```python
from build123d import *

# Parameters (mm, degrees)
F1_DEPTH = 25
F2_R     = 2.5
F3_DEPTH = 4


with BuildPart() as f1:
    # F0 (on Top) → F1 (new body)
    with BuildSketch(Plane.XY):
        with BuildLine():
            Line((-9.697168, 7.274801), (-11.697168, 7.274801))
            ThreePointArc((-11.697168, 7.274801), (-13.111381, 6.689015), (-13.697168, 5.274801))
            Line((-13.697168, 5.274801), (-13.697168, -22.725199))
            Line((-13.697168, -22.725199), (-9.697168, -22.725199))
            Line((-9.697168, -22.725199), (-9.697168, 5.024801))
            ThreePointArc((-9.697168, 5.024801), (-9.623944, 5.201578), (-9.447168, 5.274801))
            Line((-9.447168, 5.274801), (20.302832, 5.274801))
            ThreePointArc((20.302832, 5.274801), (23.278921, 2.652814), (21.052832, -0.629937))
            ThreePointArc((21.052832, -0.629937), (20.512263, -0.98581), (20.302832, -1.598182))
            ThreePointArc((20.302832, -1.598182), (20.69046, -2.388752), (21.552832, -2.566428))
            ThreePointArc((21.552832, -2.566428), (25.262981, 2.904822), (20.302832, 7.274801))
            Line((20.302832, 7.274801), (-9.697168, 7.274801))
        make_face()
    extrude(amount=F1_DEPTH)

    # F2 (on face) → F3 (cut, through all)
    with BuildSketch(Plane(origin=(-13.697168, 0, 0), x_dir=(0, -1, 0), z_dir=(-1, 0, 0))):
        with Locations((12.725199, 12.5)):
            Circle(F2_R)
    extrude(amount=-F3_DEPTH, mode=Mode.SUBTRACT)


solid = f1.part
```
Design review of the part built by this model. Coordinates are the model's own, in mm. A direction names the side the tool comes from. Coordinates: 2 decimals unless noted, no trailing zeros. Write each loop counter-clockwise with the first axis right and the second up, starting at its lowest first coordinate (ties: lowest second). Pieces come first, ordered by that corner, then holes. Notation, with made-up numbers: M -30.75,-9 L -9.75,-9 A11 ccw -9.75,6 Z; hole C -32,45 d8. An arc over 180 degrees is marked long. Answer as a JSON object with one key per item and string values.
Item 1: Draft analysis for pull direction Y (two halves, no side actions). For faces 3 (the cylindrical face through (-11.725, -13.879, 10.282)), 4 (the flat face through (5, 7.275, 12)), 5 (the flat face through (-12, -22.725, 12)), 6 (the cylindrical face through (23.27, 2.71, 12.32)), state which applies: pulls with the +Y half, pulls with the -Y half, needs draft (parallel to the pull), parting line crosses it, or undercut.
Outcome:
{"face 3": "undercut", "face 4": "pulls with the +Y half", "face 5": "pulls with the -Y half", "face 6": "undercut"}
Item 2: Add section B-B, the plane x = 22. Give the boundary of the cut face in (y, z), and give its area (3 significant figures).
Outcome:
{"outline": "M -2.43,0 L -0.2,0 L -0.2,25 L -2.43,25 Z; M 4.75,0 L 6.98,0 L 6.98,25 L 4.75,25 Z", "area": "111 mm²"}
Item 3: Add section D-D, the plane z = 21.25. Give the boundary of the cut face in (x, y), and give its area (3 significant figures).
Outcome:
{"outline": "M -13.7,-22.73 L -9.7,-22.73 L -9.7,5.02 A0.25 cw -9.45,5.27 L 20.3,5.27 A3 cw 21.05,-0.63 A1 ccw 21.55,-2.57 A5 ccw 20.3,7.27 L -11.7,7.27 A2 ccw -13.7,5.27 Z", "area": "204 mm²"}
Item 4: Insertion check: pin 1 Ø7.5 at (x, z) = (5.5, 17.5) entering from -Y; pin 2 Ø4 at (x, y) = (-9.5, -15.5) entering from +Z; pin 3 Ø1 at (y, z) = (-5.5, 13.5) entering from +X; pin 4 Ø5 at (y, z) = (-1, 9) entering from +X. Each pin has a flat end and moves straight along its axis. Give the tip position at first contact, or say it passes through.
Outcome:
{"pin 1": "y = 5.27", "pin 2": "z = 25", "pin 3": "x = -9.7", "pin 4": "x = 25.24"}
Item 5: Machinability: for faces 1 (the flat face through (-9.697, -9, 12)), 2 (the flat face through (-10, -3, 0)), which of the approach directions +Z, -Z, +X, -X, +Y, -Y give a long, thin tool a straight path to every point of the face, cutting with its end or side? Answer none if there is none.
Outcome:
{"face 1": "+Z, -Z, -Y", "face 2": "-Z, +X, -X, +Y, -Y"}
Item 6: Add section A-A, the plane z = 12.5. Give the boundary of the cut face in (x, y).
Outcome:
{"outline": "M -13.7,-22.73 L -9.7,-22.73 L -9.7,-15.23 L -13.7,-15.23 Z; M -13.7,-10.23 L -9.7,-10.23 L -9.7,5.02 A0.25 cw -9.45,5.27 L 20.3,5.27 A3 cw 21.05,-0.63 A1 ccw 21.55,-2.57 A5 ccw 20.3,7.27 L -11.7,7.27 A2 ccw -13.7,5.27 Z"}
Item 7: Wall thickness on probe 1 along Y at (x, z) = (3, 9); probe 2 along X at (y, z) = (-6, 11.5); probe 3 along X at (y, z) = (0, 19): over which ranges is each line inside the solid? List them lowest first.
Outcome:
{"probe 1": "5.27 to 7.27", "probe 2": "-13.7 to -9.7", "probe 3": "-13.7 to -9.7, 22.26 to 24.76"}
Item 8: Add section C-C, the plane y = 0.5. Give the boundary of the cut face in (x, z), and give its area (3 significant figures).
Outcome:
{"outline": "M -13.7,0 L -9.7,0 L -9.7,25 L -13.7,25 Z; M 22.72,0 L 24.98,0 L 24.98,25 L 22.72,25 Z", "area": "156 mm²"}
